Design review of the part shown in the three views and the two pictorial views. Dimensions are in mm from the part's minimum x, y and z. A direction names the side the tool comes from. Coordinates: 2 decimals unless noted, no trailing zeros. Loops run counter-clockwise (first coordinate to the right, second up) from the corner with the lowest first, then second, coordinate; pieces in that order, holes last. Notation, with made-up numbers: (-21, 77.25) -> (29, 77.25) arc R32 ccw to (29, 113.25) -> close; hole circle Ø10 at (-27, 22.25). An arc over 180 degrees is marked (long way). One line per item, written item: value.
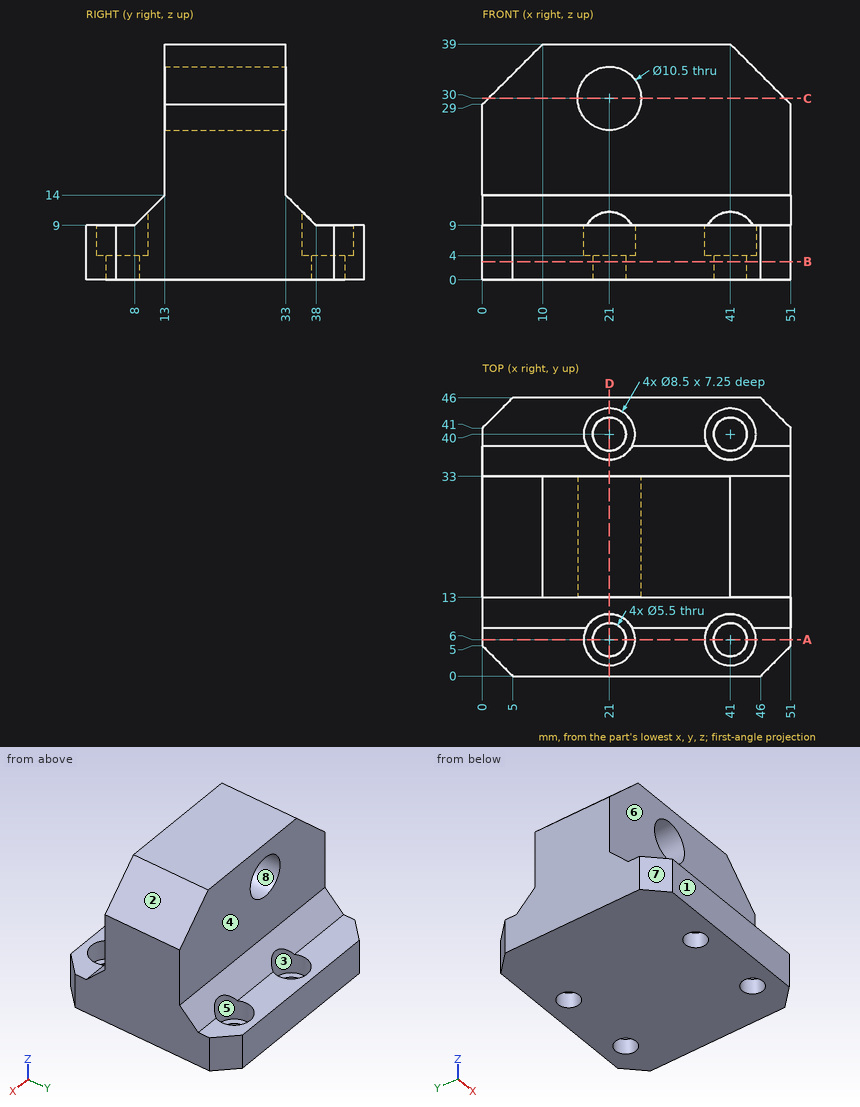
1. Insertion check: pin 1 Ø4 at (x, y) = (22.5, 42) entering from +Z; pin 2 Ø9 at (x, y) = (26.5, 4.5) entering from +Z; pin 3 Ø12 at (x, z) = (8, 21.5) entering from -Y; pin 4 Ø7 at (x, y) = (21, 6) entering from -Z. Each pin has a flat end and moves straight along its axis. Give the tip position at first contact, or say it passes through.
Return value:
pin 1: stops at z = 9
pin 2: stops at z = 10
pin 3: stops at y = 13
pin 4: stops at z = 0
2. For the marked faces 4, 5, 6, 7 and 8, list the 3-axis set-ups (+Z, -Z, +X, -X, +Y, -Y) from which the entire face can be reached by the end or side of a thin tool; tool diameter is ignored.
Return value:
face 4: +Z, +X, -X, +Y
face 5: +Z
face 6: +Z, +X, -X, -Y
face 7: +Z, -Z, -X, -Y
face 8: +Y, -Y
3. Take a section at A-A, the plane y = 6. Give the boundary of the cut face in (x, z), and give its area (3 significant figures).
Return value:
outline: (0, 0) -> (18.25, 0) -> (18.25, 4) -> (16.75, 4) -> (16.75, 9) -> (0, 9) -> close; (23.75, 0) -> (38.25, 0) -> (38.25, 4) -> (36.75, 4) -> (36.75, 9) -> (25.25, 9) -> (25.25, 4) -> (23.75, 4) -> close; (43.75, 0) -> (51, 0) -> (51, 9) -> (45.25, 9) -> (45.25, 4) -> (43.75, 4) -> close
area: 330 mm2
4. Take a section at C-C, the plane z = 30. Give the boundary of the cut face in (x, y).
Return value:
outline: (1, 13) -> (15.75, 13) -> (15.75, 33) -> (1, 33) -> close; (26.25, 13) -> (50, 13) -> (50, 33) -> (26.25, 33) -> close
5. Take a section at D-D, the plane x = 21. Give the boundary of the cut face in (y, z), and give its area (3 significant figures).
Return value:
outline: (0, 0) -> (3.25, 0) -> (3.25, 4) -> (1.75, 4) -> (1.75, 9) -> (0, 9) -> close; (8.75, 0) -> (37.25, 0) -> (37.25, 4) -> (35.75, 4) -> (35.75, 11.25) -> (33, 14) -> (33, 24.75) -> (13, 24.75) -> (13, 14) -> (10.25, 11.25) -> (10.25, 4) -> (8.75, 4) -> close; (13, 35.25) -> (33, 35.25) -> (33, 39) -> (13, 39) -> close; (42.75, 0) -> (46, 0) -> (46, 9) -> (44.25, 9) -> (44.25, 4) -> (42.75, 4) -> close
area: 695 mm2
6. To check wall thickness, follow probe 1 along X at (y, z) = (6, 1); probe 2 along Y at (x, z) = (41, 2.2); probe 3 along X at (y, z) = (40, 7). State the ranges of each line that lie inside material, in increasing order. Write a range as from..to.
Return value:
probe 1: x = 0..18.25, 23.75..38.25, 43.75..51
probe 2: y = 0..3.25, 8.75..37.25, 42.75..46
probe 3: x = 0..16.75, 25.25..36.75, 45.25..51
7. The part is to be moulded in two halves that separate along X. For the marked faces 1, 2 and 3, say which applies: pulls with the +X half, pulls with the -X half, needs draft (parallel to the pull), parting line crosses it, or undercut.
Return value:
face 1: needs draft
face 2: pulls with the +X half
face 3: undercut
8. Take a section at B-B, the plane z = 3. Give the boundary of the cut face in (x, y), and give its area (3 significant figures).
Return value:
outline: (0, 5) -> (5, 0) -> (46, 0) -> (51, 5) -> (51, 41) -> (46, 46) -> (5, 46) -> (0, 41) -> close; hole circle Ø5.5 at (21, 6); hole circle Ø5.5 at (21, 40); hole circle Ø5.5 at (41, 6); hole circle Ø5.5 at (41, 40)
area: 2,200 mm2
